Check sheet for the modelled part. Datum: model origin and axes. Units: mm. A direction names the side the tool comes from. Coordinates: 2 decimals unless noted, no trailing zeros. Loops run counter-clockwise (first coordinate to the right, second up) from the corner with the lowest first, then second, coordinate; pieces in that order, holes last. Notation, with made-up numbers: (77.5, 33) - (88.5, 33) arc R18 ccw to (88.5, 55) - close; hole circle Ø3 at (-1.5, 58). An arc over 180 degrees is marked (long way). Use a Markdown table: item, result. Add a question column.
1) Draft check along Y on faces 1 (the cylindrical face through (10.14, -7.73, 72.5)), 2 (the flat face through (10, 0, 50)), 3 (the flat face through (0, -2, 31)). Enter one of: pulls with the +Y half, pulls with the -Y half, needs draft (parallel to the pull), parting line crosses it, or undercut.
2) Tool access check on faces 4 (the flat face through (10, 17, 20)), 5 (the flat face through (10, 35, 10)). Record the directions out of +Z, -Z, +X, -X, +Y, -Y that give a thin tool (end or side, any length) a straight path to the whole face; none if there is none.
3) Go/stop test with flat-tipped pins: P1, Ø2, axis at x = 6, y = 27, coming from the +Z side; P2, Ø1.5, axis at x = 15.5, z = 29.5, coming from the +Y side; P3, Ø7, axis at y = -12.5, z = 26, coming from the +X side. Record where each tip stops, or that it passes through.
4) Sectioned sample at C-C, the plane x = 11.75. Enter the section's corners in (y, z).
5) Sectioned sample at D-D, the plane z = 26. Enter the section's corners in (x, y), then the cut area to 3 significant figures.
6) Thickness scan on line 1 (Z direction, x = 4.5, y = -12.5); line 2 (Y direction, x = 10.75, z = 61); line 3 (Y direction, x = 10.5, z = 37.5). Record the ranges inside material, lowest first.
7) Sectioned sample at B-B, the plane y = -12.5. Enter the section's corners in (x, z).
8) Sectioned sample at A-A, the plane z = 71. Enter the section's corners in (x, y).
from build123d import *

# Parameters (mm, degrees)
F0_W     = 20
F0_H     = 25
F1_DEPTH = 80
F2_R     = 5
F2_R_2   = 4.5
F3_DEPTH = 25
F4_W     = 20
F4_H     = 20
F5_DEPTH = 35


with BuildPart() as f1:
    # F0 (on Top) → F1 (new body)
    with BuildSketch(Plane.XY):
        with Locations((10, -12.5)):
            Rectangle(F0_W, F0_H)
    extrude(amount=F1_DEPTH)

    # F2 (on face) → F3 (cut)
    with BuildSketch(Plane.YZ.offset(20)):
        with Locations((-12.5, 71)):
            Circle(F2_R)
        with Locations((-12.5, 56)):
            Circle(F2_R_2)
        with Locations((-12.5, 41)):
            Circle(F2_R)
        with Locations((-12.5, 26)):
            Circle(F2_R_2)
    extrude(amount=-F3_DEPTH, mode=Mode.SUBTRACT)

    # F4 (on face) → F5 (join)
    with BuildSketch(Plane(origin=(0, 0, 0), x_dir=(-1, 0, 0), z_dir=(0, 1, 0))):
        with Locations((-10, 10)):
            Rectangle(F4_W, F4_H)
    extrude(amount=F5_DEPTH)


solid = f1.part
Solved:
| question | item | result |
|---|---|---|
| 1 | face 1 | undercut |
| 1 | face 2 | pulls with the +Y half |
| 1 | face 3 | needs draft |
| 2 | face 4 | +Z, +X, -X, +Y |
| 2 | face 5 | +Z, -Z, +X, -X, +Y |
| 3 | P1 | stops at z = 20 |
| 3 | P2 | stops at y = 0 |
| 3 | P3 | passes through |
| 4 | outline | (-25, 0) - (35, 0) - (35, 20) - (0, 20) - (0, 80) - (-25, 80) - close; hole circle Ø10 at (-12.5, 41); hole circle Ø10 at (-12.5, 71); hole circle Ø9 at (-12.5, 26); hole circle Ø9 at (-12.5, 56) |
| 5 | outline | (0, -25) - (20, -25) - (20, -17) - (0, -17) - close; (0, -8) - (20, -8) - (20, 0) - (0, 0) - close |
| 5 | area | 320 mm2 |
| 6 | line 1 | z = 0 to 21.5, 30.5 to 36, 46 to 51.5, 60.5 to 66, 76 to 80 |
| 6 | line 2 | y = -25 to 0 |
| 6 | line 3 | y = -25 to -16.07, -8.93 to 0 |
| 7 | outline | (0, 0) - (20, 0) - (20, 21.5) - (0, 21.5) - close; (0, 30.5) - (20, 30.5) - (20, 36) - (0, 36) - close; (0, 46) - (20, 46) - (20, 51.5) - (0, 51.5) - close; (0, 60.5) - (20, 60.5) - (20, 66) - (0, 66) - close; (0, 76) - (20, 76) - (20, 80) - (0, 80) - close |
| 8 | outline | (0, -25) - (20, -25) - (20, -17.5) - (0, -17.5) - close; (0, -7.5) - (20, -7.5) - (20, 0) - (0, 0) - close |
